from build123d import *

# Parameters (mm, degrees)
BOSS_EXTRUDE1_DEPTH          = 25.4
SKETCH3_W                    = 25.4
SKETCH3_H                    = 6.35
BOSS_EXTRUDE3_DEPTH          = 38.1
CUT_EXTRUDE1_START           = 5.08
CUT_EXTRUDE1_DEPTH           = 3.556
CUT_EXTRUDE1_DRAFT           = 2
CUT_EXTRUDE1_PROFILE_2_DEPTH = 3.556
CUT_EXTRUDE1_PROFILE_2_DRAFT = 2
CUT_EXTRUDE1_PROFILE_3_DEPTH = 3.556
CUT_EXTRUDE1_PROFILE_3_DRAFT = 2
CUT_EXTRUDE1_PROFILE_4_DEPTH = 3.556
CUT_EXTRUDE1_PROFILE_4_DRAFT = 2
CUT_EXTRUDE1_PROFILE_5_DEPTH = 3.556
CUT_EXTRUDE1_PROFILE_5_DRAFT = 2
CUT_EXTRUDE1_PROFILE_6_DEPTH = 3.556
CUT_EXTRUDE1_PROFILE_6_DRAFT = 2


with BuildPart() as part:
    # Sketch1 → Boss-Extrude1 (new body)
    with BuildSketch(Plane(origin=(0, 0, 0), x_dir=(1, 0, 0), z_dir=(0, 1, 0))):
        with BuildLine():
            Line((-1.27, 3.89197217), (1.27, 3.89197217))
            Line((1.27, 3.89197217), (1.27, 2.315656298))
            ThreePointArc((1.27, 2.315656298), (0, -2.641053595), (-1.27, 2.315656298))
            Line((-1.27, 2.315656298), (-1.27, 3.89197217))
        make_face()
    extrude(amount=BOSS_EXTRUDE1_DEPTH)

    # Sketch3 → Boss-Extrude3 (add)
    with BuildSketch(Plane(origin=(0, 0, -3.89197217), x_dir=(-1, 0, 0), z_dir=(0, 0, -1))):
        with Locations((0, 18.011112495)):
            Rectangle(SKETCH3_W, SKETCH3_H)
    extrude(amount=BOSS_EXTRUDE3_DEPTH)


with BuildPart() as cut_extrude1_tool:
    # Sketch4 → Cut-Extrude1 (with draft: the straight prism first)
    with BuildSketch(Plane.XY.offset(CUT_EXTRUDE1_START)):
        Polygon((-3.113495219, 25.001271063), (-3.113495219, 23.121671063), (2.876409327, 22.06548928), (2.876409327, 23.94508928), align=None)
    extrude(amount=-CUT_EXTRUDE1_DEPTH)
    # Cut-Extrude1: the draft: its side faces are tilted about the plane it starts from
    cut_extrude1_sides = [cut_extrude1_tool.faces().sort_by_distance(p)[0] for p in [
        (-3.113495219, 24.061471063, 3.302),
        (-0.118542946, 22.593580171, 3.302),
        (2.876409327, 23.00528928, 3.302),
        (-0.118542946, 24.473180171, 3.302),
    ]]
    draft(cut_extrude1_sides, Plane.XY.offset(CUT_EXTRUDE1_START), CUT_EXTRUDE1_DRAFT)


with BuildPart() as part_1:
    add(part.part)

    # Cut-Extrude1: cut by cut_extrude1_tool
    add(cut_extrude1_tool.part, mode=Mode.SUBTRACT)


with BuildPart() as cut_extrude1_profile_2_tool:
    # Sketch4 → Cut-Extrude1 profile 2 (with draft: the straight prism first)
    with BuildSketch(Plane.XY.offset(CUT_EXTRUDE1_START)):
        Polygon((-3.113495219, 16.670071063), (-3.113495219, 14.790471063), (2.876409327, 13.73428928), (2.876409327, 15.61388928), align=None)
    extrude(amount=-CUT_EXTRUDE1_PROFILE_2_DEPTH)
    # Cut-Extrude1 profile 2: the draft: its side faces are tilted about the plane it starts from
    cut_extrude1_profile_2_sides = [cut_extrude1_profile_2_tool.faces().sort_by_distance(p)[0] for p in [
        (-3.113495219, 15.730271063, 3.302),
        (-0.118542946, 14.262380171, 3.302),
        (2.876409327, 14.67408928, 3.302),
        (-0.118542946, 16.141980171, 3.302),
    ]]
    draft(cut_extrude1_profile_2_sides, Plane.XY.offset(CUT_EXTRUDE1_START), CUT_EXTRUDE1_PROFILE_2_DRAFT)


with BuildPart() as part_2:
    add(part_1.part)

    # Cut-Extrude1 profile 2: cut by cut_extrude1_profile_2_tool
    add(cut_extrude1_profile_2_tool.part, mode=Mode.SUBTRACT)


with BuildPart() as cut_extrude1_profile_3_tool:
    # Sketch4 → Cut-Extrude1 profile 3 (with draft: the straight prism first)
    with BuildSketch(Plane.XY.offset(CUT_EXTRUDE1_START)):
        Polygon((-3.113495219, 20.835671063), (-3.113495219, 18.956071063), (2.876409327, 17.89988928), (2.876409327, 19.77948928), align=None)
    extrude(amount=-CUT_EXTRUDE1_PROFILE_3_DEPTH)
    # Cut-Extrude1 profile 3: the draft: its side faces are tilted about the plane it starts from
    cut_extrude1_profile_3_sides = [cut_extrude1_profile_3_tool.faces().sort_by_distance(p)[0] for p in [
        (-3.113495219, 19.895871063, 3.302),
        (-0.118542946, 18.427980171, 3.302),
        (2.876409327, 18.83968928, 3.302),
        (-0.118542946, 20.307580171, 3.302),
    ]]
    draft(cut_extrude1_profile_3_sides, Plane.XY.offset(CUT_EXTRUDE1_START), CUT_EXTRUDE1_PROFILE_3_DRAFT)


with BuildPart() as part_3:
    add(part_2.part)

    # Cut-Extrude1 profile 3: cut by cut_extrude1_profile_3_tool
    add(cut_extrude1_profile_3_tool.part, mode=Mode.SUBTRACT)


with BuildPart() as cut_extrude1_profile_4_tool:
    # Sketch4 → Cut-Extrude1 profile 4 (with draft: the straight prism first)
    with BuildSketch(Plane.XY.offset(CUT_EXTRUDE1_START)):
        Polygon((-3.113495219, 12.504471063), (-3.113495219, 10.624871063), (2.876409327, 9.56868928), (2.876409327, 11.44828928), align=None)
    extrude(amount=-CUT_EXTRUDE1_PROFILE_4_DEPTH)
    # Cut-Extrude1 profile 4: the draft: its side faces are tilted about the plane it starts from
    cut_extrude1_profile_4_sides = [cut_extrude1_profile_4_tool.faces().sort_by_distance(p)[0] for p in [
        (-3.113495219, 11.564671063, 3.302),
        (-0.118542946, 10.096780171, 3.302),
        (2.876409327, 10.50848928, 3.302),
        (-0.118542946, 11.976380171, 3.302),
    ]]
    draft(cut_extrude1_profile_4_sides, Plane.XY.offset(CUT_EXTRUDE1_START), CUT_EXTRUDE1_PROFILE_4_DRAFT)


with BuildPart() as part_4:
    add(part_3.part)

    # Cut-Extrude1 profile 4: cut by cut_extrude1_profile_4_tool
    add(cut_extrude1_profile_4_tool.part, mode=Mode.SUBTRACT)


with BuildPart() as cut_extrude1_profile_5_tool:
    # Sketch4 → Cut-Extrude1 profile 5 (with draft: the straight prism first)
    with BuildSketch(Plane.XY.offset(CUT_EXTRUDE1_START)):
        Polygon((-3.113495219, 8.338871063), (-3.113495219, 6.459271063), (2.876409327, 5.40308928), (2.876409327, 7.28268928), align=None)
    extrude(amount=-CUT_EXTRUDE1_PROFILE_5_DEPTH)
    # Cut-Extrude1 profile 5: the draft: its side faces are tilted about the plane it starts from
    cut_extrude1_profile_5_sides = [cut_extrude1_profile_5_tool.faces().sort_by_distance(p)[0] for p in [
        (-3.113495219, 7.399071063, 3.302),
        (-0.118542946, 5.931180171, 3.302),
        (2.876409327, 6.34288928, 3.302),
        (-0.118542946, 7.810780171, 3.302),
    ]]
    draft(cut_extrude1_profile_5_sides, Plane.XY.offset(CUT_EXTRUDE1_START), CUT_EXTRUDE1_PROFILE_5_DRAFT)


with BuildPart() as part_5:
    add(part_4.part)

    # Cut-Extrude1 profile 5: cut by cut_extrude1_profile_5_tool
    add(cut_extrude1_profile_5_tool.part, mode=Mode.SUBTRACT)


with BuildPart() as cut_extrude1_profile_6_tool:
    # Sketch4 → Cut-Extrude1 profile 6 (with draft: the straight prism first)
    with BuildSketch(Plane.XY.offset(CUT_EXTRUDE1_START)):
        Polygon((-3.113495219, 4.173271063), (-3.113495219, 2.293671063), (2.876409327, 1.23748928), (2.876409327, 3.11708928), align=None)
    extrude(amount=-CUT_EXTRUDE1_PROFILE_6_DEPTH)
    # Cut-Extrude1 profile 6: the draft: its side faces are tilted about the plane it starts from
    cut_extrude1_profile_6_sides = [cut_extrude1_profile_6_tool.faces().sort_by_distance(p)[0] for p in [
        (-3.113495219, 3.233471063, 3.302),
        (-0.118542946, 1.765580171, 3.302),
        (2.876409327, 2.17728928, 3.302),
        (-0.118542946, 3.645180171, 3.302),
    ]]
    draft(cut_extrude1_profile_6_sides, Plane.XY.offset(CUT_EXTRUDE1_START), CUT_EXTRUDE1_PROFILE_6_DRAFT)


with BuildPart() as part_6:
    add(part_5.part)

    # Cut-Extrude1 profile 6: cut by cut_extrude1_profile_6_tool
    add(cut_extrude1_profile_6_tool.part, mode=Mode.SUBTRACT)


solid = part_6.part
For this review, take the finished solid that the model builds, in its own axes (mm). A direction names the side the tool comes from. Give positions to 0.01 mm unless a question says otherwise; leave off trailing zeros. Order: outer loops, then holes, each group sorted by start corner. A loop starts at its lowest first (then second) coordinate and runs counter-clockwise, first axis right, second up. Notation, with made-up numbers: M 39,25.5 L 65,25.5 A16 cw 65,33.5 Z; hole C 20,14 d3. An arc over 180 degrees is marked long. Answer in a Markdown table with one row per item. Add a question column.
(1) Wall thickness on probe 1 along Y at (x, z) = (-0.5, -7.5); probe 2 along Z at (x, y) = (8.25, 19.5); probe 3 along Z at (x, y) = (1.75, 18.75): over which ranges is each line inside the solid? List them lowest first. Write a range as [from, to].
(2) For faces 4 (the face through (0, 23, -3.892)), 5 (the face through (0, 18, -41.992)), list the 3-axis set-ups (+Z, -Z, +X, -X, +Y, -Y) from which the entire face can be reached by the end or side of a thin tool; tool diameter is ignored.
(3) Mouldability with a two-part tool opening along Z and no side actions: class faces 1 (the face through (0, 25.4, -1)), 2 (the face through (0, 7, -3.892)), 3 (the face through (-1.27, 13, -3)) as +Z half, -Z half, draft (parallel to the pull), parting line (faces both ways), or undercut.
(4) Consider section C-C on x = 10.25. State the section outline as (y, z) points, and give its area (3 significant figures).
(5) For pin 1 (2.5 mm diameter, centred on x = 0.5, y = 3.5, fed in from +Z); pin 2 (3 mm diameter, centred on x = 6, y = 17.5, fed in from +Z); pin 3 (12.5 mm diameter, centred on x = -2.5, z = -21.5, fed in from -Y); pin 4 (1.5 mm diameter, centred on x = -0.5, z = -26, fed in from +Y), all flat-tipped, find the tip position at first contact; note any pin that passes through.
(6) Consider section A-A on z = -11. State the section outline as (x, y) points.
Evaluation:
| question | item | result |
|---|---|---|
| 1 | probe 1 | y = [14.84, 21.19] |
| 1 | probe 2 | z = [-41.99, -3.89] |
| 1 | probe 3 | z = [-41.99, -3.89], [-1.98, 1.52] |
| 2 | face 4 | -Z, +X, -X, +Y |
| 2 | face 5 | -Z, +X, -X, +Y, -Y |
| 3 | face 1 | draft |
| 3 | face 2 | -Z half |
| 3 | face 3 | undercut |
| 4 | outline | M 14.84,-41.99 L 21.19,-41.99 L 21.19,-3.89 L 14.84,-3.89 Z |
| 4 | area | 242 mm^2 |
| 5 | pin 1 | stops at z = 2.64 |
| 5 | pin 2 | stops at z = -3.89 |
| 5 | pin 3 | stops at y = 14.84 |
| 5 | pin 4 | stops at y = 21.19 |
| 6 | outline | M -12.7,14.84 L 12.7,14.84 L 12.7,21.19 L -12.7,21.19 Z |
